Source: three-view drawing plus pictorial views. Frame: mm from the lowest corner of the part. A direction names the side the tool comes from. Give positions to 0.01 mm unless a question says otherwise; leave off trailing zeros. Order: outer loops, then holes, each group sorted by start corner. A loop starts at its lowest first (then second) coordinate and runs counter-clockwise, first axis right, second up. Notation, with made-up numbers: (6, 11.5) - (63, 11.5) arc R8 ccw to (63, 17.5) - close; hole circle Ø6 at (51, 34). An arc over 180 degrees is marked (long way). Answer in a Markdown table with one row per item. Add a question column.
1. Section query D-D on x = 11.5. Return loops of the section in (y, z) (1 decimal).
2. Section query C-C on x = 25. Return loops of the section in (y, z) (1 decimal).
3. Section query A-A on z = 3. Return loops of the section in (x, y) (1 decimal), and give its area (3 significant figures).
4. Ray query, line 1 (Y direction, x = 25.5, z = 4.75) (1 decimal); line 2 (Y direction, x = 22, z = 4.5) (1 decimal); line 3 (Z direction, x = 8.5, y = 6.5) (1 decimal). Return the intervals inside material, ascending. Write a range as [from, to].
5. Access query for the marked faces 5 and 6. Directions: +Z, -Z, +X, -X, +Y, -Y. A direction counts if a zero-diameter tool reaches every point of the face in a straight line with its end or side. Return the directions, or none.
6. Contact query for flat-ended pins moving along their axis: pin 1 (1 mm diameter, centred on y = 32, z = 1.5, fed in from -X); pin 2 (4 mm diameter, centred on y = 16.5, z = 7.5, fed in from -X) (1 decimal); pin 3 (1.5 mm diameter, centred on y = 12.5, z = 6, fed in from +X). Output: stop coordinate, or through.
7. Mould query, pull axis X, two halves, no side actions, for the marked faces 1, 2, 3 and 4. Classes: released by +X, released by -X, zero draft, split by the parting line, or undercut.
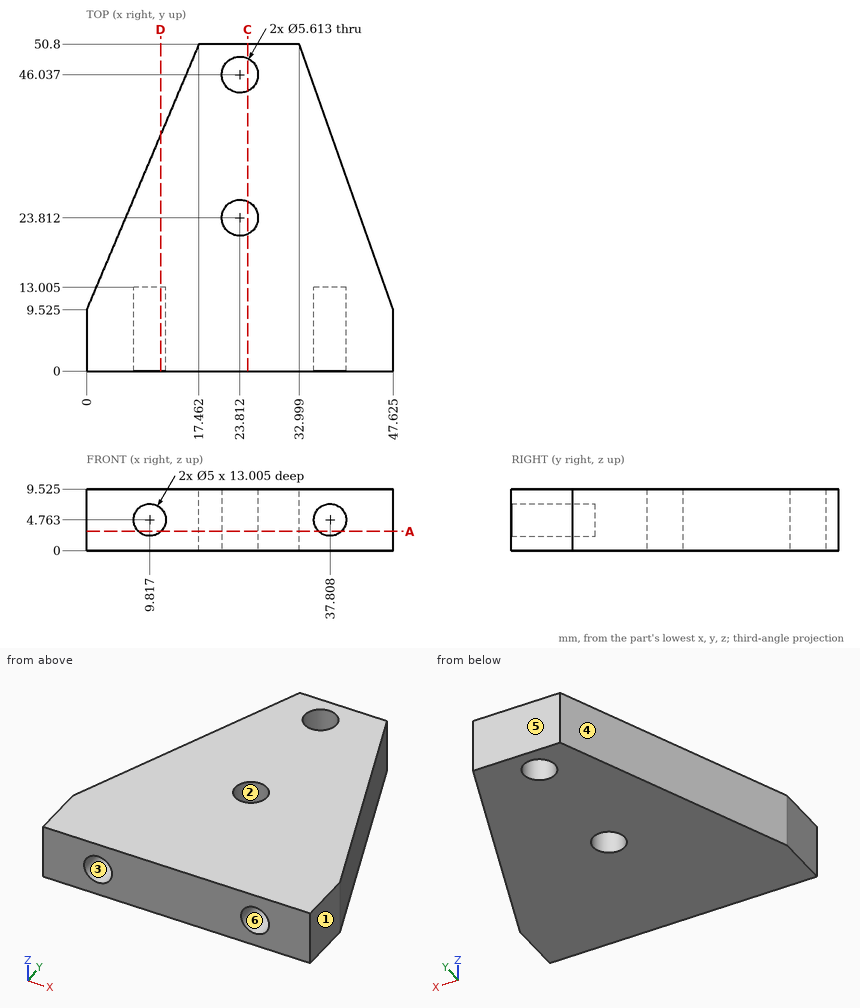
Answer:
| question | item | result |
|---|---|---|
| 1 | outline | (0, 0) - (36.7, 0) - (36.7, 9.5) - (0, 9.5) - (0, 6.6) - (13, 6.6) - (13, 2.9) - (0, 2.9) - close |
| 2 | outline | (0, 0) - (21.3, 0) - (21.3, 9.5) - (0, 9.5) - close; (26.4, 0) - (43.5, 0) - (43.5, 9.5) - (26.4, 9.5) - close; (48.6, 0) - (50.8, 0) - (50.8, 9.5) - (48.6, 9.5) - close |
| 3 | outline | (0, 0) - (8, 0) - (8, 13) - (11.6, 13) - (11.6, 0) - (36, 0) - (36, 13) - (39.6, 13) - (39.6, 0) - (47.6, 0) - (47.6, 9.5) - (33, 50.8) - (17.5, 50.8) - (0, 9.5) - close; hole circle Ø5.6 at (23.8, 23.8); hole circle Ø5.6 at (23.8, 46) |
| 3 | area | 1,620 mm² |
| 4 | line 1 | y = [0, 21.6], [26.1, 43.8], [48.3, 50.8] |
| 4 | line 2 | y = [0, 21.7], [26, 43.9], [48.2, 50.8] |
| 4 | line 3 | z = [0, 2.6], [6.9, 9.5] |
| 5 | face 5 | +Z, -Z, +X, -X, +Y |
| 5 | face 6 | -Y |
| 6 | pin 1 | stops at x = 9.3 |
| 6 | pin 2 | stops at x = 2.1 |
| 6 | pin 3 | stops at x = 46.84 |
| 7 | face 1 | released by +X |
| 7 | face 2 | undercut |
| 7 | face 3 | undercut |
| 7 | face 4 | released by -X |
